Autodesk Inventor part; units mm, degrees
ref_plane "YZ Plane" through (0, 0, 0) normal (1, 0, 0) x (0, 1, 0)
ref_plane "XZ Plane" through (0, 0, 0) normal (0, 1, 0) x (-1, 0, 0)
ref_plane "XY Plane" through (0, 0, 0) normal (0, 0, 1) x (1, 0, 0)
sketch "Náčrt1" plane through (0, 0, 0) normal (0, 1, 0) x (-1, 0, 0)
  line L0 (0, 0) -> (-150, 0)
  line L1 (-150, 0) -> (-150, -100)
  line L2 (-150, -100) -> (0, -100)
  line L3 (0, -100) -> (0, 0)
  dimension "d0" = 150
  dimension "d1" = 100
extrude "Vysunutí1" add sketch "Náčrt1" along normal blind 1.5
fillet "Zaoblení1" radius 10 4 edges at (150, 0.75, -100) (150, 0.75, 0) (0, 0.75, 0) (0, 0.75, -100)
sketch "Náčrt3" plane through (0, 1.5, 0) normal (0, 1, 0) x (1, 0, 0)
  line L0 (3.5, 96.5) -> (146.5, 96.5)
  line L1 (146.5, 96.5) -> (146.5, 3.5)
  line L2 (146.5, 3.5) -> (3.5, 3.5)
  line L3 (3.5, 3.5) -> (3.5, 96.5)
  line L4 (0, 90) -> (0, 10)
  line L5 (10, 0) -> (140, 0)
  point P0 (0, 0)
  dimension "d11" = 3.5
  dimension "d12" = 3.5
  dimension "d13" = 93
  dimension "d14" = 143
extrude "Vysunutí3" add sketch "Náčrt3" along normal blind 25
sketch "Náčrt4" plane through (0, 26.5, 0) normal (0, 1, 0) x (1, 0, 0)
  line L0 (3.5, 96.5) -> (3.5, 3.5)
  line L1 (5.5, 94.5) -> (144.5, 94.5)
  line L2 (144.5, 94.5) -> (144.5, 5.5)
  line L3 (144.5, 5.5) -> (5.5, 5.5)
  line L4 (5.5, 5.5) -> (5.5, 94.5)
  line L5 (3.5, 3.5) -> (146.5, 3.5)
  point P0 (0, 0)
  point P1 (3.5, 13.5)
  point P2 (13.5, 3.5)
  point P3 (136.5, 3.5)
  dimension "d19" = 2
  dimension "d20" = 2
  dimension "d21" = 139
  dimension "d22" = 89
extrude "Vysunutí4" cut sketch "Náčrt4" against normal blind 25
fillet "Zaoblení3" radius 10 8 edges at (144.5, 14, -94.5) (5.5, 14, -94.5) (5.5, 14, -5.5) (144.5, 14, -5.5) (3.5, 14, -96.5) (3.5, 14, -3.5) (146.5, 14, -96.5) (146.5, 14, -3.5)
sketch "Náčrt5" plane through (13.5, 1.5, -3.5) normal (0, 0, 1) x (1, 0, 0)
  line L0 (121, 25) -> (2, 25)
  line L1 (133, 0) -> (133, 25)
  line L2 (-10, 25) -> (-10, 0)
  line L3 (121, 0) -> (121, 25)
  line L4 (2, 25) -> (2, 0)
  line L5 (121, 3) -> (2, 3)
  line L6 (2, 3) -> (2, 25)
  line L7 (2, 25) -> (121, 25)
  line L8 (121, 25) -> (121, 3)
  point P0 (-13.5, -1.5)
extrude "Vysunutí5" cut sketch "Náčrt5" against normal blind 2
sketch "Náčrt6" plane through (136.5, 1.5, -96.5) normal (0, 0, -1) x (-1, 0, 0)
  line L0 (121, 25) -> (2, 25)
  line L1 (76, 25) -> (62, 25)
  line L2 (62, 25) -> (62, 20)
  line L3 (62, 20) -> (76, 20)
  line L4 (76, 20) -> (76, 25)
  line L5 (53, 25) -> (41, 25)
  line L6 (41, 25) -> (41, 20)
  line L7 (41, 20) -> (53, 20)
  line L8 (53, 20) -> (53, 25)
  line L9 (123, 25) -> (123, 0)
  line L10 (0, 0) -> (0, 25)
  point P0 (136.5, -1.5)
  point P1 (41, 25)
  dimension "d30" = 47
  dimension "d31" = 61
  dimension "d32" = 41
  dimension "d33" = 53
  dimension "d34" = 5
extrude "Vysunutí6" cut sketch "Náčrt6" against normal blind 2
properties part number "víko"
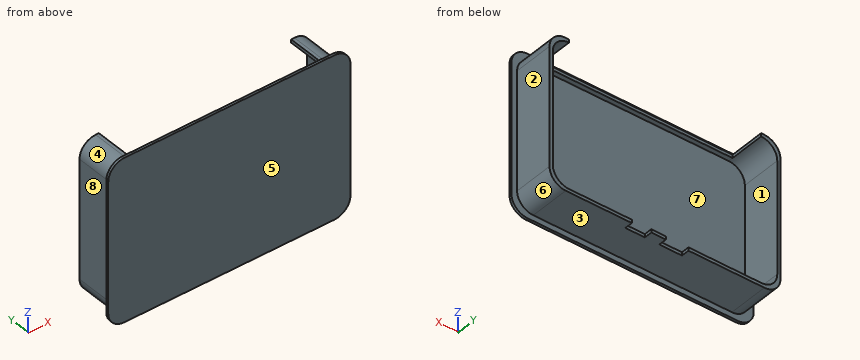
Could you check a few things on this model? Use its own coordinates, in mm. Face numbers are marked on the shaded views. A direction names the side the tool comes from. Give positions to 0.01 mm unless a question says otherwise; leave off trailing zeros. Loops run counter-clockwise (first coordinate to the right, second up) from the corner with the lowest first, then second, coordinate; pieces in that order, holes last. Notation, with made-up numbers: M 1.5,-16.75 L 35.5,-16.75 A24 ccw 35.5,22.25 Z; hole C 20.25,55.25 d7. An arc over 180 degrees is marked long. Answer as a JSON object with one key per item and string values.
Q1. Suppose I cut it at C-C, the plane x = 133. List the corners of the cut face in (y, z) for me, plus the area to 3 significant figures.
Values found:
{"outline": "M 0,-100 L 1.5,-100 L 1.5,-96.5 L 26.5,-96.5 L 26.5,-94.5 L 1.5,-94.5 L 1.5,-5.5 L 4.5,-5.5 L 4.5,-3.5 L 1.5,-3.5 L 1.5,0 L 0,0 Z", "area": "206 mm²"}
Q2. If I drill on probe 1 along X at (y, z) = (12, -49); probe 2 along Z at (x, y) = (27, 13.75); probe 3 along Y at (x, z) = (144, -58), over which ranges is the centre line in solid material (lowest first)? Write a range as [from, to].
Values found:
{"probe 1": "x = [3.5, 5.5], [144.5, 146.5]", "probe 2": "z = [-96.5, -94.5]", "probe 3": "y = [0, 1.5]"}
Q3. For the marked faces 1, 2, 3, 4 and 5, which set-ups out of +Z, -Z, +X, -X, +Y, -Y let a thin tool reach every point of the face, with its end or its side?
Values found:
{"face 1": "+Y", "face 2": "+Z, -Z, +X, +Y", "face 3": "-Z, +X, -X, +Y", "face 4": "+Z, -X, +Y", "face 5": "+Z, -Z, +X, -X, -Y"}
Q4. Suppose I cut it at B-B, the plane z = -56.5. List the corners of the cut face in (x, y) for me.
Values found:
{"outline": "M 0,0 L 150,0 L 150,1.5 L 146.5,1.5 L 146.5,26.5 L 144.5,26.5 L 144.5,1.5 L 5.5,1.5 L 5.5,26.5 L 3.5,26.5 L 3.5,1.5 L 0,1.5 Z"}
Q5. For P1, Ø2, axis at y = 20.5, z = -32.5, coming from the -X side; P2, Ø1, axis at y = 23.5, z = -96, coming from the -X side; P3, Ø12, axis at y = 9.5, z = -11, coming from the +X side, each with a flat end and sliding along its axis, tell me the tip position at first contact or that it passes through.
Values found:
{"P1": "stops at x = 3.5", "P2": "stops at x = 9.14", "P3": "stops at x = 146.5"}
Q6. Suppose I cut it at A-A, the plane y = 24.25. List the corners of the cut face in (x, z) for me.
Values found:
{"outline": "M 3.5,-86.5 A10 ccw 13.5,-96.5 L 60.5,-96.5 L 60.5,-94.5 L 15.5,-94.5 A10 cw 5.5,-84.5 L 5.5,-15.5 A10 cw 15.5,-5.5 L 15.5,-3.5 L 13.5,-3.5 A10 ccw 3.5,-13.5 Z; M 74.5,-96.5 L 83.5,-96.5 L 83.5,-94.5 L 74.5,-94.5 Z; M 95.5,-96.5 L 136.5,-96.5 A10 ccw 146.5,-86.5 L 146.5,-13.5 A10 ccw 136.5,-3.5 L 134.5,-3.5 L 134.5,-5.5 A10 cw 144.5,-15.5 L 144.5,-84.5 A10 cw 134.5,-94.5 L 95.5,-94.5 Z"}
Q7. If we mould it in two halves opening along X, with no side actions, what happens to the marked faces 6, 7 and 8? For each: pulls with the +X half, pulls with the -X half, needs draft (parallel to the pull), parting line crosses it, or undercut.
Values found:
{"face 6": "pulls with the +X half", "face 7": "undercut", "face 8": "pulls with the -X half"}
